Here's the drawing with two shaded views (mm, measured from the low corner). I have some questions. A direction names the side the tool comes from. Round coordinates to 2 decimals unless told otherwise and drop trailing zeros. Order: outer loops, then holes, each group sorted by start corner. A loop starts at its lowest first (then second) coordinate and runs counter-clockwise, first axis right, second up. Notation, with made-up numbers: (41, 7) - (57, 7) arc R20 cw to (57, 21) - close; hole circle Ø6 at (89.5, -36). An arc over 180 degrees is marked (long way). One line per item, written item: value.
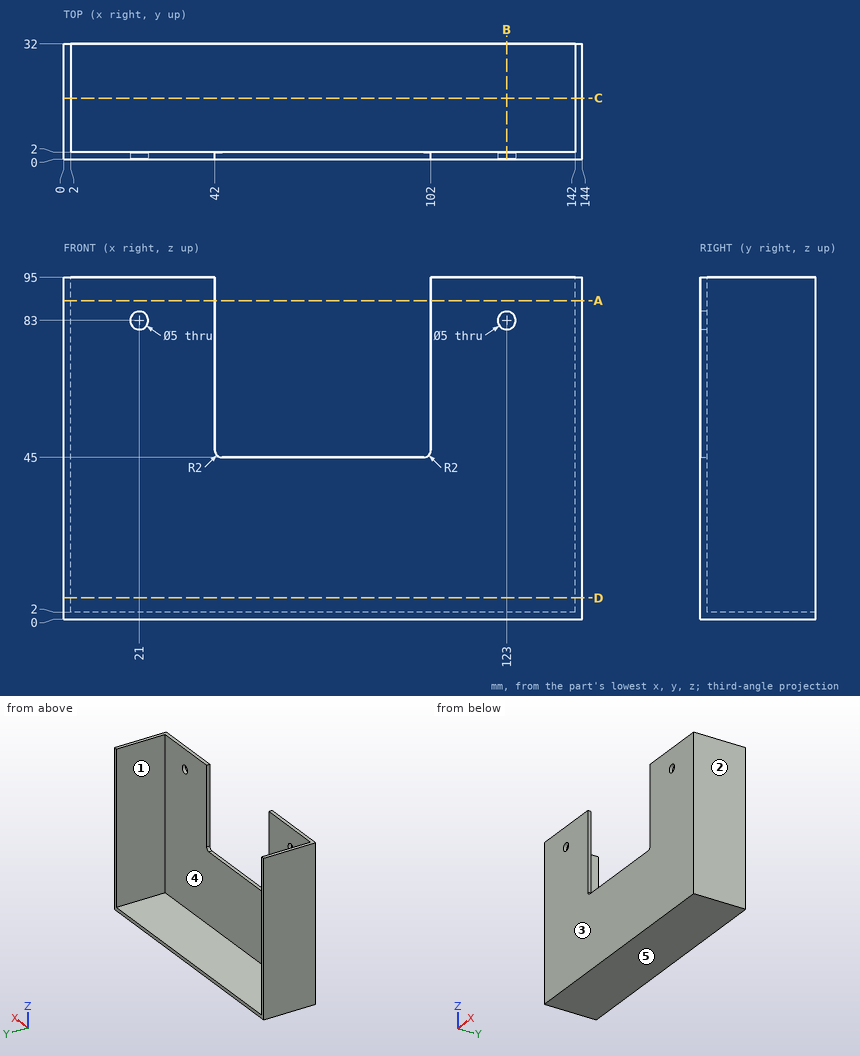
Q1. We'd pull the mould along X, two halves only. Please class the marked faces 1, 2 and 3: released by +X, released by -X, zero draft, split by the parting line, or undercut.
Results list:
face 1: undercut
face 2: released by +X
face 3: zero draft
Q2. Which directions (+Z, -Z, +X, -X, +Y, -Y) give clear straight access to the entire face, cutting with the end or side of a thin tool? Please do the marked faces 4 and 5.
Results list:
face 4: +Z, +Y
face 5: -Z, +X, -X, +Y, -Y
Q3. Will these pins go through, and if not, where does the flat tip stop? pin 1 (8 mm diameter, centred on x = 26.5, z = 66.5, fed in from +Y); pin 2 (1 mm diameter, centred on x = 71, y = 1, fed in from +Z).
Results list:
pin 1: y = 2
pin 2: z = 45
Q4. If we section it at A-A, the plane z = 88.5: Please give me the cut outline in (x, y).
Results list:
outline: (0, 0) - (42, 0) - (42, 2) - (2, 2) - (2, 32) - (0, 32) - close; (102, 0) - (144, 0) - (144, 32) - (142, 32) - (142, 2) - (102, 2) - close
Q5. If we section it at B-B, the plane x = 123: Please give me the cut outline in (y, z), then the cut area to 3 significant figures.
Results list:
outline: (0, 0) - (32, 0) - (32, 2) - (2, 2) - (2, 80.5) - (0, 80.5) - close; (0, 85.5) - (2, 85.5) - (2, 95) - (0, 95) - close
area: 240 mm²
Q6. If I drill on line 1 along X through (y, z) = (1.4, 83); line 2 along X through (y, z) = (19.5, 22.5); line 3 along Z through (x, y) = (123, 1), over which ranges is the centre line in solid material (lowest first)?
Results list:
line 1: 0 to 18.5, 23.5 to 42, 102 to 120.5, 125.5 to 144
line 2: 0 to 2, 142 to 144
line 3: 0 to 80.5, 85.5 to 95
Q7. If we section it at D-D, the plane z = 6: Please give me the cut outline in (x, y), then the cut area to 3 significant figures.
Results list:
outline: (0, 0) - (144, 0) - (144, 32) - (142, 32) - (142, 2) - (2, 2) - (2, 32) - (0, 32) - close
area: 408 mm²
Q8. If we section it at C-C, the plane y = 17: Please give me the cut outline in (x, z), then the cut area to 3 significant figures.
Results list:
outline: (0, 0) - (144, 0) - (144, 95) - (142, 95) - (142, 2) - (2, 2) - (2, 95) - (0, 95) - close
area: 660 mm²
